from build123d import *

# Parameters (mm, degrees)
SKETCH1_W             = 20
SKETCH1_H             = 20
BOSS_EXTRUDE1_DEPTH   = 100
M5_CLEARANCE_HOLE1_D  = 5.5
M5_TAPPED_HOLE3_D     = 4.2
M5_TAPPED_HOLE3_DEPTH = 10.4
M5_TAPPED_HOLE3_TIP   = 1.2618073


with BuildPart() as part:
    # Sketch1 → Boss-Extrude1 (new body)
    with BuildSketch(Plane(origin=(0, 0, 0), x_dir=(1, 0, 0), z_dir=(0, 1, 0))):
        with Locations((10, 10)):
            Rectangle(SKETCH1_W, SKETCH1_H)
    extrude(amount=BOSS_EXTRUDE1_DEPTH)

    # Sketch5 → M8 Tapped Hole1 (revolve, cut)
    with BuildSketch(Plane(origin=(10, 100, -10), x_dir=(0, 0, 1), z_dir=(1, 0, 0))):
        Polygon((0, 0), (0, 15.792926105), (3.4, 13.75), (3.4, 0), align=None)
    m8_tapped_hole1 = revolve(axis=Axis((10, 106.35, -10), (0, -1, 0)), mode=Mode.SUBTRACT)

    # Mirror1: M8 Tapped Hole1 across plane
    add(m8_tapped_hole1.mirror(Plane.ZX.offset(50)), mode=Mode.SUBTRACT)

    # M5 Clearance Hole1 (through all)
    with Locations(Plane(origin=(20, 0, 0), x_dir=(0, 0, -1), z_dir=(1, 0, 0))):
        with Locations((10, 20), (10, 80)):
            Hole(M5_CLEARANCE_HOLE1_D / 2)

    # M5 Tapped Hole3
    with Locations(Plane(origin=(20, 0, 0), x_dir=(0, 0, -1), z_dir=(1, 0, 0))):
        with Locations((10, 92.5)):
            Hole(M5_TAPPED_HOLE3_D / 2, depth=M5_TAPPED_HOLE3_DEPTH)
            with Locations((0, 0, -(M5_TAPPED_HOLE3_DEPTH + M5_TAPPED_HOLE3_TIP / 2))):  # 118° drill point
                Cone(0, M5_TAPPED_HOLE3_D / 2, M5_TAPPED_HOLE3_TIP, mode=Mode.SUBTRACT)


solid = part.part
For this review, take the finished solid that the model builds, in its own axes (mm). A direction names the side the tool comes from. Give positions to 0.01 mm unless a question says otherwise; leave off trailing zeros. Loops run counter-clockwise (first coordinate to the right, second up) from the corner with the lowest first, then second, coordinate; pieces in that order, holes last. Notation, with made-up numbers: M -36,84 L 17,84 A9 cw 17,94 Z; hole C -3,-9.75 d9. An arc over 180 degrees is marked long. Answer as a JSON object with one key per item and string values. Group by question number.
Q1. Add section A-A on x = 16. Give the boundary of the cut face in (y, z).
Q2. Insertion check: P1, Ø8, axis at x = 10, z = -10, coming from the +Y side; P2, Ø3.5, axis at y = 80, z = -10, coming from the -X side (1 decimal). Each pin has a flat end and moves straight along its axis. Give the tip position at first contact, or say it passes through.
Q3. For probe 1 along Y at (x, z) = (14.5, -10); probe 2 along Y at (x, z) = (10.25, -12); probe 3 along Y at (x, z) = (1.25, -10.25), list the stretches that pass through material, from the lowest coordinate up. Write a range as [from, to].
Q4. Tool access review of faces 5 (the cylindrical face through (16.29, 92.59, -12.1)), 6 (the cylindrical face through (13.32, 6.78, -10.74)), 7 (the cylindrical face through (6.63, 93.22, -10.44)): name each direction out of +Z, -Z, +X, -X, +Y, -Y from which nothing blocks a thin tool from reaching the whole face with its end or side.
Q5. Add section B-B on y = 80. Give the boundary of the cut face in (x, z).
Q6. Add section D-D on y = 92.5. Give the boundary of the cut face in (x, z).
Q7. Add section C-C on x = 3. Give the boundary of the cut face in (y, z).
Q8. Mouldability with a two-part tool opening along X and no side actions: class faces 1 (the flat face through (0, 49, -10)), 2 (the cylindrical face through (9.86, 80.83, -7.38)), 3 (the flat face through (20, 49, -10)), 4 (the conical face through (9.82, 84.56, -9.44)) as +X half, -X half, draft (parallel to the pull), parting line (faces both ways), or undercut.
Checked values:
{
 "1": {"outline": "M 0,-20 L 100,-20 L 100,0 L 0,0 Z; hole C 20,-10 d5.5; hole C 80,-10 d5.5; hole C 92.5,-10 d4.2"},
 "2": {"P1": "y = 100", "P2": "through"},
 "3": {"probe 1": "[0, 17.25], [22.75, 77.25], [82.75, 90.4], [94.6, 100]", "probe 2": "[14.58, 18.11], [21.89, 78.11], [81.89, 85.42]", "probe 3": "[0, 17.26], [22.74, 77.26], [82.74, 100]"},
 "4": {"face 5": "+X", "face 6": "-Y", "face 7": "+Y"},
 "5": {"outline": "M 0,-20 L 20,-20 L 20,-12.75 L 0,-12.75 Z; M 0,-7.25 L 20,-7.25 L 20,0 L 0,0 Z"},
 "6": {"outline": "M 0,-20 L 20,-20 L 20,-12.1 L 12.67,-12.1 A3.4 cw long 12.67,-7.9 L 20,-7.9 L 20,0 L 0,0 Z"},
 "7": {"outline": "M 0,-20 L 100,-20 L 100,0 L 0,0 Z; hole C 20,-10 d5.5; hole C 80,-10 d5.5"},
 "8": {"face 1": "-X half", "face 2": "draft", "face 3": "+X half", "face 4": "undercut"}
}
